from build123d import *

# Parameters (mm, degrees)
SKETCH_R     = 8.5
SKETCH_R_2   = 3
PAD_DEPTH    = 4
SKETCH001_R  = 8.5
PAD001_DEPTH = 5
CHAMFER_SIZE = 0.5


with BuildPart() as part:
    # Sketch → Pad (new body)
    with BuildSketch(Plane.XY):
        Circle(SKETCH_R)
        Circle(SKETCH_R_2, mode=Mode.SUBTRACT)
    extrude(amount=PAD_DEPTH)

    # Sketch001 (on Face4 of Pad) → Pad001 (join)
    with BuildSketch(Plane.XY.offset(4)):
        Circle(SKETCH001_R)
        Polygon((6.5, -3.752777), (6.5, 3.752777), (0, 7.505553), (-6.5, 3.752777), (-6.5, -3.752777), (0, -7.505553), align=None, mode=Mode.SUBTRACT)
    extrude(amount=PAD001_DEPTH)

    # Chamfer
    chamfer_edges = [part.edges().sort_by_distance(p)[0] for p in [
        (-3.25, 5.629165, 9),
        (3.25, 5.629165, 9),
        (6.5, 0, 9),
        (3.25, -5.629165, 9),
        (-3.25, -5.629165, 9),
        (-6.5, 0, 9),
    ]]
    chamfer(chamfer_edges, length=CHAMFER_SIZE)


solid = part.part
The listing builds one solid part. Answer for the finished solid, in the listing's coordinates (mm). A direction names the side the tool comes from. Round coordinates to 2 decimals unless told otherwise and drop trailing zeros. Order: outer loops, then holes, each group sorted by start corner. A loop starts at its lowest first (then second) coordinate and runs counter-clockwise, first axis right, second up. Notation, with made-up numbers: (60.25, 88) -> (104.25, 88) arc R23 cw to (104.25, 125) -> close; hole circle Ø6 at (36.5, 61.25). An arc over 180 degrees is marked (long way). Write each question's results on one line, items separated by ' | '. Start each with the question number.
Q1. The mould has two halves that part along X. Classify faces 1 (the cylindrical face through (4.57, 7.167, 4.437)), 2 (the flat face through (3.2, -5.66, 6.22)), 3 (the flat face through (4, 0, 0)): pulls with the +X half, pulls with the -X half, needs draft (parallel to the pull), parting line crosses it, or undercut.
Q2. Which of the six approach directions +Z, -Z, +X, -X, +Y, -Y give full straight-line access (tool end or side, diameter ignored) to faces 4 (the flat face through (-0.1, -3.2, 4)), 5 (the cylindrical face through (-3, 0, 2))?
Q3. Find section C-C (x = -2.25). Determine the outline of the cut face in (y, z), then the cut area to 3 significant figures.
Q4. Find section A-A (y = 0). Determine the outline of the cut face in (x, z), then the cut area to 4 significant figures.
Q5. Each of these flat-tipped pins is pushed along its axis until it touches: pin 1 (2 mm diameter, centred on x = -2, y = 2, fed in from -Z); pin 2 (3 mm diameter, centred on x = 4.5, z = 3, fed in from -Y); pin 3 (7 mm diameter, centred on x = 0, y = 0, fed in from +Z); pin 4 (3 mm diameter, centred on x = -6, z = 2, fed in from +Y). Where does it stop, or does it pass through?
Q6. Find section D-D (x = 5). Determine the outline of the cut face in (y, z), then the cut area to 3 significant figures.
Q7. Straight lines are drawn through the part: probe 1 along Y at (x, z) = (0, 1.45); probe 2 along X at (y, z) = (-2.5, 1.5); probe 3 along X at (y, z) = (-4, 5). For each, find the intervals that lie inside material, in ascending order. Write a range as from..to.
Q8. Find section B-B (z = 7.5). Determine the outline of the cut face in (x, y), then the cut area to 3 significant figures.
Worked answers:
1) face 1: parting line crosses it | face 2: undercut | face 3: needs draft
2) face 4: +Z | face 5: +Z, -Z
3) outline: (-8.2, 0) -> (-1.98, 0) -> (-1.98, 4) -> (-6.21, 4) -> (-6.21, 8.5) -> (-6.78, 9) -> (-8.2, 9) -> close; (1.98, 0) -> (8.2, 0) -> (8.2, 9) -> (6.78, 9) -> (6.21, 8.5) -> (6.21, 4) -> (1.98, 4) -> close | area: 69.3 mm2
4) outline: (-8.5, 0) -> (-3, 0) -> (-3, 4) -> (-6.5, 4) -> (-6.5, 8.5) -> (-7, 9) -> (-8.5, 9) -> close; (3, 0) -> (8.5, 0) -> (8.5, 9) -> (7, 9) -> (6.5, 8.5) -> (6.5, 4) -> (3, 4) -> close | area: 63.75 mm2
5) pin 1: stops at z = 0 | pin 2: stops at y = -7.95 | pin 3: stops at z = 4 | pin 4: stops at y = 7.21
6) outline: (-6.87, 0) -> (6.87, 0) -> (6.87, 9) -> (5.2, 9) -> (4.62, 8.5) -> (4.62, 4) -> (-4.62, 4) -> (-4.62, 8.5) -> (-5.2, 9) -> (-6.87, 9) -> close | area: 77.3 mm2
7) probe 1: y = -8.5..-3, 3..8.5 | probe 2: x = -8.12..-1.66, 1.66..8.12 | probe 3: x = -7.5..-6.07, 6.07..7.5
8) outline: circle Ø17 at (0, 0); hole (-6.5, -3.75) -> (0, -7.51) -> (6.5, -3.75) -> (6.5, 3.75) -> (0, 7.51) -> (-6.5, 3.75) -> close | area: 80.6 mm2
